Source: CAD feature listing. Evaluate the final solid. Frame: model axes, mm. A direction names the side the tool comes from. Round coordinates to 2 decimals unless told otherwise and drop trailing zeros. Loops run counter-clockwise (first coordinate to the right, second up) from the corner with the lowest first, then second, coordinate; pieces in that order, holes last.
Item 1: First-contact query: P1, Ø1.5, axis at y = 95.5, z = 60.5, coming from the -X side; P2, Ø10.5, axis at x = -1.5, z = 40.5, coming from the -Y side; P3, Ø2.5, axis at y = 109, z = 62, coming from the +X side. Flat tips, straight axial feed; report the tip coordinate or a pass-through.
Item 2: Access query for faces 1 (the flat face through (-3, 26, 62)), 2 (the cylindrical face through (-1.08, 140.93, -4.88)), 3 (the flat face through (-10, 132, 24)), 4 (the cylindrical face through (-1.08, -21.8, -4.88)), 5 (the flat face through (0, 128, 31)). Directions: +Z, -Z, +X, -X, +Y, -Y. A direction counts if a zero-diameter tool reaches every point of the face in a straight line with its end or side. Return the directions, or none.
Item 3: Section query A-A on x = 0. Give the number of separate pieces and of enclosed holes in the cut face, then the cut area to 3 significant figures.
Item 4: Section query D-D on x = -13. Return loops of the section in (y, z).
Item 5: Pull-direction query (X, two-part tool) for faces 6 (the cylindrical face through (0, 6, 62)), 7 (the cylindrical face through (18.152, 36.468, 61.513)), 8 (the cylindrical face through (0.25, -6.5, 62.62)); classes: released by +X, released by -X, zero draft, split by the parting line, or undercut.
Item 6: Section query C-C on z = 43.5. Return loops of the section in (x, y), then the cut area to 3 significant figures.
Item 7: Section query B-B on y = 64. Return loops of the section in (x, z).
Item 8: Ray query, L1, parallel to X at y = 64, z = 60.6; L2, parallel to Y at x = -3, z = 6; L3, parallel to Y at x = 0, z = 60.35. Return the intervals inside material, ascending.
```python
from build123d import *

# Parameters (mm, degrees)
SKETCH1_W             = 144
SKETCH1_H             = 35
BOSS_EXTRUDE1_DEPTH   = 5
BOSS_EXTRUDE2_DEPTH   = 8
FILLET1_R             = 10
BOSS_EXTRUDE3_DEPTH   = 8
SKETCH5_R             = 5
BOSS_EXTRUDE4_DEPTH   = 28
FILLET1_OF_MIRROR1_R  = 10
FILLET3_R             = 5
SKETCH7_R             = 2.5
CUT_EXTRUDE2_DEPTH    = 28
SKETCH8_R             = 5
CUT_EXTRUDE3_DEPTH    = 18
SKETCH9_W             = 50
SKETCH9_H             = 4.833302034
BOSS_EXTRUDE7_DEPTH   = 5
FILLET6_R             = 5
FILLET7_R             = 5
SKETCH10_W            = 50
SKETCH10_H            = 5
BOSS_EXTRUDE8_DEPTH   = 5
FILLET8_R             = 5
FILLET9_R             = 5
CUT_EXTRUDE6_DEPTH    = 10
BODY_MOVE_COPY1_ANGLE = 120


with BuildPart() as part:
    # Sketch1 → Boss-Extrude1 (new body)
    with BuildSketch(Plane(origin=(0, 0, 0), x_dir=(1, 0, 0), z_dir=(0, 1, 0))):
        Rectangle(SKETCH1_W, SKETCH1_H)
    boss_extrude1 = extrude(amount=BOSS_EXTRUDE1_DEPTH)

    # Sketch3 → Boss-Extrude2 (add)
    with BuildSketch(Plane.ZY.offset(72)):
        Polygon((-17.5, 5), (-17.5, 15), (-10, 15), (-10, 55), (10, 55), (10, 15), (17.5, 15), (17.5, 5), (0, 5), align=None)
    boss_extrude2 = extrude(amount=-BOSS_EXTRUDE2_DEPTH)

    # Fillet1
    # the kernel refuses this fillet: 10 mm, written as the material it takes off along each edge
    with BuildSketch(Plane(origin=(-96.206145914, 15, -17.5), x_dir=(0, -1, 0), z_dir=(1, 0, 0))) as fillet1_piece_1:
        with BuildLine():
            CenterArc((9.682458366, -10), FILLET1_R, 90, 75.522487814)
            Line((0, -7.5), (-0.193649167, -7.45))
            ThreePointArc((-0.193649167, -7.45), (-0.2, -3.75), (-0.2, 0))
            Line((-0.2, 0), (0, 0.2))
            Line((0, 0.2), (9.682458366, 0.2))
            Line((9.682458366, 0.2), (9.682458366, 0))
        make_face()
    extrude(amount=56.412291828, mode=Mode.SUBTRACT)
    with BuildSketch(Plane(origin=(-96.206145914, 15, 17.5), x_dir=(0, -1, 0), z_dir=(1, 0, 0))) as fillet1_piece_2:
        with BuildLine():
            CenterArc((9.682458366, 10), FILLET1_R, 194.477512186, 75.522487814)
            Line((0, 7.5), (-0.193649167, 7.45))
            ThreePointArc((-0.193649167, 7.45), (-0.2, 3.75), (-0.2, 0))
            Line((-0.2, 0), (0, -0.2))
            Line((0, -0.2), (9.682458366, -0.2))
            Line((9.682458366, -0.2), (9.682458366, 0))
        make_face()
    extrude(amount=56.412291828, mode=Mode.SUBTRACT)

    # Sketch4 → Boss-Extrude3 (add)
    with BuildSketch(Plane.ZY.offset(72)):
        with BuildLine():
            Line((-10, 55), (-10, 65))
            ThreePointArc((-10, 65), (0, 75), (10, 65))
            Line((10, 65), (10, 55))
            Line((10, 55), (-10, 55))
        make_face()
    boss_extrude3 = extrude(amount=-BOSS_EXTRUDE3_DEPTH)

    # Sketch5 → Boss-Extrude4 (add)
    with BuildSketch(Plane.ZY.offset(72)):
        with Locations(Location((0, 64.047898896, 0), (0, 0, 180))):
            Circle(SKETCH5_R)
    boss_extrude4 = extrude(amount=BOSS_EXTRUDE4_DEPTH)

    # Mirror1: Boss-Extrude1, Boss-Extrude2, Boss-Extrude3, Boss-Extrude4 across plane
    add(boss_extrude1.mirror(Plane(origin=(0, 0, 0), x_dir=(0, 0, 1), z_dir=(1, 0, 0))))
    add(boss_extrude2.mirror(Plane(origin=(0, 0, 0), x_dir=(0, 0, 1), z_dir=(1, 0, 0))))
    add(boss_extrude3.mirror(Plane(origin=(0, 0, 0), x_dir=(0, 0, 1), z_dir=(1, 0, 0))))
    add(boss_extrude4.mirror(Plane(origin=(0, 0, 0), x_dir=(0, 0, 1), z_dir=(1, 0, 0))))

    # Fillet1 of Mirror1
    # the kernel refuses this fillet: 10 mm, written as the material it takes off along each edge
    with BuildSketch(Plane(origin=(96.206145914, 15, -17.5), x_dir=(0, -1, 0), z_dir=(-1, 0, 0))) as fillet1_of_mirror1_piece_1:
        with BuildLine():
            CenterArc((9.682458366, 10), FILLET1_OF_MIRROR1_R, 194.477512186, 75.522487814)
            Line((0, 7.5), (-0.193649167, 7.45))
            ThreePointArc((-0.193649167, 7.45), (-0.2, 3.75), (-0.2, 0))
            Line((-0.2, 0), (0, -0.2))
            Line((0, -0.2), (9.682458366, -0.2))
            Line((9.682458366, -0.2), (9.682458366, 0))
        make_face()
    extrude(amount=56.412291828, mode=Mode.SUBTRACT)
    with BuildSketch(Plane(origin=(96.206145914, 15, 17.5), x_dir=(0, -1, 0), z_dir=(-1, 0, 0))) as fillet1_of_mirror1_piece_2:
        with BuildLine():
            CenterArc((9.682458366, -10), FILLET1_OF_MIRROR1_R, 90, 75.522487814)
            Line((0, -7.5), (-0.193649167, -7.45))
            ThreePointArc((-0.193649167, -7.45), (-0.2, -3.75), (-0.2, 0))
            Line((-0.2, 0), (0, 0.2))
            Line((0, 0.2), (9.682458366, 0.2))
            Line((9.682458366, 0.2), (9.682458366, 0))
        make_face()
    extrude(amount=56.412291828, mode=Mode.SUBTRACT)

    # Fillet3
    fillet3_edges = [part.edges().sort_by_distance(p)[0] for p in [
        (-72, 0, 0),
        (72, 0, 0),
    ]]
    fillet(fillet3_edges, radius=FILLET3_R)

    # Sketch7 → Cut-Extrude2 (cut)
    with BuildSketch(Plane(origin=(0, 5, 0), x_dir=(1, 0, 0), z_dir=(0, 1, 0))):
        with Locations(Location((0, 0, 0), (0, 0, 270))):
            Circle(SKETCH7_R)
    extrude(amount=-CUT_EXTRUDE2_DEPTH, mode=Mode.SUBTRACT)

    # Sketch8 → Cut-Extrude3 (cut)
    with BuildSketch(Plane(origin=(100, 0, 0), x_dir=(0, 0, -1), z_dir=(1, 0, 0))):
        with Locations(Location((0, 64.047898896, 0), (0, 0, 180))):
            Circle(SKETCH8_R)
    extrude(amount=-CUT_EXTRUDE3_DEPTH, mode=Mode.SUBTRACT)

    # Sketch9 → Boss-Extrude7 (add)
    with BuildSketch(Plane.XZ):
        with Locations((0.833489832, 19.916651017)):
            Rectangle(SKETCH9_W, SKETCH9_H)
    extrude(amount=-BOSS_EXTRUDE7_DEPTH)

    # Fillet6
    # the kernel refuses this fillet: 5 mm, written as the material it adds along each edge
    with BuildSketch(Plane(origin=(-24.166510168, 0, 17.5), x_dir=(-1, 0, 0), z_dir=(0, 1, 0))) as fillet6_piece_1:
        with BuildLine():
            CenterArc((4.997220406, 5), FILLET6_R, 181.91057204, 88.08942796)
            Line((0, 4.833302034), (-0.099944408, 4.829968074))
            ThreePointArc((-0.099944408, 4.829968074), (-0.1, 2.416651017), (-0.1, 0))
            Line((-0.1, 0), (0, -0.1))
            Line((0, -0.1), (4.997220406, -0.1))
            Line((4.997220406, -0.1), (4.997220406, 0))
        make_face()
    extrude(amount=5)
    with BuildSketch(Plane(origin=(25.833489832, 0, 17.5), x_dir=(1, 0, 0), z_dir=(0, 1, 0))) as fillet6_piece_2:
        with BuildLine():
            CenterArc((4.997220406, -5), FILLET6_R, 90, 88.08942796)
            Line((0, -4.833302034), (-0.099944408, -4.829968074))
            ThreePointArc((-0.099944408, -4.829968074), (-0.1, -2.416651017), (-0.1, 0))
            Line((-0.1, 0), (0, 0.1))
            Line((0, 0.1), (4.997220406, 0.1))
            Line((4.997220406, 0.1), (4.997220406, 0))
        make_face()
    extrude(amount=5)

    # Fillet7
    fillet7_edges = [part.edges().sort_by_distance(p)[0] for p in [
        (-24.166510168, 2.5, 22.333302034),
        (25.833489832, 2.5, 22.333302034),
    ]]
    fillet(fillet7_edges, radius=FILLET7_R)

    # Sketch10 → Boss-Extrude8 (add)
    with BuildSketch(Plane.XZ):
        with Locations((0, -20)):
            Rectangle(SKETCH10_W, SKETCH10_H)
    extrude(amount=-BOSS_EXTRUDE8_DEPTH)

    # Fillet8
    fillet8_edges = [part.edges().sort_by_distance(p)[0] for p in [
        (-25, 2.5, -17.5),
        (25, 2.5, -17.5),
    ]]
    fillet(fillet8_edges, radius=FILLET8_R - 0.0001)  # a hair under: the kernel refuses the full size

    # Fillet9
    fillet9_edges = [part.edges().sort_by_distance(p)[0] for p in [
        (-25, 2.5, -22.5),
        (25, 2.5, -22.5),
    ]]
    fillet(fillet9_edges, radius=FILLET9_R)

    # Sketch11 → Cut-Extrude6 (cut)
    with BuildSketch(Plane(origin=(0, 5, 0), x_dir=(1, 0, 0), z_dir=(0, 1, 0))):
        with BuildLine():
            Line((55, -3), (20, -3))
            ThreePointArc((20, -3), (17, 0), (20, 3))
            Line((20, 3), (55, 3))
            ThreePointArc((55, 3), (58, 0), (55, -3))
        make_face()
        with BuildLine():
            Line((-55, -3), (-20, -3))
            ThreePointArc((-20, -3), (-17, 0), (-20, 3))
            Line((-20, 3), (-55, 3))
            ThreePointArc((-55, 3), (-58, 0), (-55, -3))
        make_face()
    extrude(amount=-CUT_EXTRUDE6_DEPTH, mode=Mode.SUBTRACT)


with BuildPart() as part_1:
    # Body-Move/Copy1: read off the stored shape, not the designer's step
    # Body-Move/Copy1: moved
    add(part.part.moved(Location((64, -64.0478989, 0))).rotate(Axis((0, 0, 0), (-0.5773502692, -0.5773502692, 0.5773502692)), BODY_MOVE_COPY1_ANGLE))


solid = part_1.part
```
Data:
1. P1: stops at x = -17.5
1. P2: stops at y = -8
1. P3: stops at x = 17.5
2. face 1: +Z, -Z
2. face 2: +Y
2. face 3: -Z, -X, +Y, -Y
2. face 4: -Y
2. face 5: -Z, +X, -X
3. separate pieces: 4
3. enclosed holes: 0
3. area: 1,770 mm2
4. outline: (-8, 50.38) - (0, 50.38) - (0, 59.05) - (128, 59.05) - (128, 50.38) - (136, 50.38) - (136, 59.05) arc R5 ccw to (131, 64.05) - (-3, 64.05) arc R5 ccw to (-8, 59.05) - close
5. face 6: undercut
5. face 7: released by +X
5. face 8: zero draft
6. outline: (-10, -8) - (10, -8) - (10, 0) - (-10, 0) - close; (-10, 128) - (10, 128) - (10, 136) - (-10, 136) - close
6. area: 320 mm2
7. outline: (-22.33, 59.05) - (-2.5, 59.05) - (-2.5, 64.05) - (-22.33, 64.05) - close; (2.5, 59.05) - (22.5, 59.05) - (22.5, 64.05) - (2.5, 64.05) - close
8. L1: x = -22.33 to -2.5, 2.5 to 22.5
8. L2: y = -8 to 0, 128 to 136
8. L3: y = -7.83 to 6, 47 to 61.5, 66.5 to 81, 122 to 135.83
